```python
from build123d import *

# Parameters (mm, degrees)
SKETCH1_W           = 76.2
SKETCH1_H           = 76.2
SKETCH1_R           = 3.175
BOSS_EXTRUDE1_DEPTH = 6.35
SKETCH2_W           = 28.575
SKETCH2_H           = 76.2
SKETCH2_R           = 3.175
BOSS_EXTRUDE3_DEPTH = 9.525
SKETCH4_W           = 12.7
SKETCH4_H           = 25.4
CUT_EXTRUDE1_DEPTH  = 28.575
SKETCH5_W           = 12.7
SKETCH5_H           = 32.4
CUT_EXTRUDE2_DEPTH  = 9.525
SKETCH6_R           = 1
CUT_EXTRUDE3_DEPTH  = 6.35
SKETCH7_W           = 12.7
SKETCH7_H           = 3.5
SKETCH7_R           = 1
BOSS_EXTRUDE4_DEPTH = 11.43


with BuildPart() as part:
    # Sketch1 → Boss-Extrude1 (new body)
    with BuildSketch(Plane.XY):
        Rectangle(SKETCH1_W, SKETCH1_H)
        with Locations((-28.575, 19.525)):
            Circle(SKETCH1_R, mode=Mode.SUBTRACT)
        with Locations((28.575, 19.525)):
            Circle(SKETCH1_R, mode=Mode.SUBTRACT)
        with Locations((28.575, -19.525)):
            Circle(SKETCH1_R, mode=Mode.SUBTRACT)
        with Locations((-28.575, -19.525)):
            Circle(SKETCH1_R, mode=Mode.SUBTRACT)
    extrude(amount=BOSS_EXTRUDE1_DEPTH)

    # Sketch2 → Boss-Extrude3 (add)
    with BuildSketch(Plane(origin=(0, 0, 0), x_dir=(-1, 0, 0), z_dir=(0, 0, -1))):
        with Locations((-23.8125, 0)):
            Rectangle(SKETCH2_W, SKETCH2_H)
        with Locations((-28.575, -19.525)):
            Circle(SKETCH2_R, mode=Mode.SUBTRACT)
        with Locations((-28.575, 19.525)):
            Circle(SKETCH2_R, mode=Mode.SUBTRACT)
        with Locations((23.8125, 0)):
            Rectangle(SKETCH2_W, SKETCH2_H)
        with Locations((28.575, -19.525)):
            Circle(SKETCH2_R, mode=Mode.SUBTRACT)
        with Locations((28.575, 19.525)):
            Circle(SKETCH2_R, mode=Mode.SUBTRACT)
    extrude(amount=BOSS_EXTRUDE3_DEPTH)

    # Sketch4 → Cut-Extrude1 (cut)
    with BuildSketch(Plane.ZY.offset(-9.525)):
        Rectangle(SKETCH4_W, SKETCH4_H)
    extrude(amount=-CUT_EXTRUDE1_DEPTH, mode=Mode.SUBTRACT)

    # Sketch5 → Cut-Extrude2 (cut)
    with BuildSketch(Plane(origin=(0, 0, -9.525), x_dir=(-1, 0, 0), z_dir=(0, 0, -1))):
        with Locations((-19.05, 0)):
            Rectangle(SKETCH5_W, SKETCH5_H)
    extrude(amount=-CUT_EXTRUDE2_DEPTH, mode=Mode.SUBTRACT)

    # Sketch6 → Cut-Extrude3 (cut)
    with BuildSketch(Plane(origin=(0, 0, 0), x_dir=(-1, 0, 0), z_dir=(0, 0, -1))):
        with Locations((-19.05, 14.45)):
            Circle(SKETCH6_R)
        with Locations((-19.05, -14.45)):
            Circle(SKETCH6_R)
    extrude(amount=-CUT_EXTRUDE3_DEPTH, mode=Mode.SUBTRACT)

    # Sketch7 → Boss-Extrude4 (add)
    with BuildSketch(Plane(origin=(0, 0, 0), x_dir=(-1, 0, 0), z_dir=(0, 0, -1))):
        with Locations((-19.05, -14.45)):
            Rectangle(SKETCH7_W, SKETCH7_H)
        with Locations((-19.05, -14.45)):
            Circle(SKETCH7_R, mode=Mode.SUBTRACT)
        with Locations((-19.05, 14.45)):
            Rectangle(SKETCH7_W, SKETCH7_H)
        with Locations((-19.05, 14.45)):
            Circle(SKETCH7_R, mode=Mode.SUBTRACT)
    extrude(amount=BOSS_EXTRUDE4_DEPTH)


solid = part.part
```
Here's how the part is built. I have some questions about the finished solid (model axes, mm). A direction names the side the tool comes from. Coordinates: 2 decimals unless noted, no trailing zeros. Write each loop counter-clockwise with the first axis right and the second up, starting at its lowest first coordinate (ties: lowest second). Pieces come first, ordered by that corner, then holes. Notation, with made-up numbers: (13.5, 54) -> (45.5, 54) arc R15 ccw to (45.5, 59) -> close; hole circle Ø4 at (-33, -24). An arc over 180 degrees is marked (long way). Use a Markdown table: item, result. Add a question column.
(1) I'm going to push flat-ended pins straight in: P1, Ø1.5, axis at y = -14.5, z = -11, coming from the -X side; P2, Ø0.6, axis at x = 16.5, z = -10.5, coming from the -Y side; P3, Ø8.5, axis at x = 28.575, y = -19.525, coming from the -Z side (3 decimals). Where does each tip first touch, or does it pass through?
(2) For faces 1 (the flat face through (12.7, 14, -10)), 2 (the flat face through (32, 0, -6.35)), 3 (the flat face through (19, -16.2, -10)), 4 (the flat face through (25.4, 14, -10)), which set-ups out of +Z, -Z, +X, -X, +Y, -Y let a thin tool reach every point of the face, with its end or its side?
(3) Please list where these lines run through material, in increasing order: line 1 (Y direction, x = 19.05, z = -4); line 2 (Y direction, x = -28.5, z = 2.25); line 3 (Y direction, x = 14, z = 0.25).
(4) If we section it at D-D, the plane y = -14.45: Write out the boundary of the cut face in (x, z) (3 decimals).
(5) We'd pull the mould along Y, two halves only. Please class faces 5 (the flat face through (-9.525, -1, -5)), 6 (the flat face through (19, 16.2, -10)), 7 (the flat face through (25.4, 0, -8)): +Y half, -Y half, draft (parallel to the pull), parting line (faces both ways), or undercut.
(6) If we section it at C-C, the plane x = 19.05: Write out the boundary of the cut face in (y, z) (3 decimals), and give its area (3 significant figures).
(7) If we section it at B-B, the plane y = 5.5: Write out the boundary of the cut face in (x, z) (3 decimals), and give its area (3 significant figures).
(8) If we section it at A-A, the plane z = -10.5: Write out the boundary of the cut face in (x, y).
Outcome:
| question | item | result |
|---|---|---|
| 1 | P1 | stops at x = 12.7 |
| 1 | P2 | stops at y = -16.2 |
| 1 | P3 | stops at z = -9.525 |
| 2 | face 1 | -Z, -X, +Y, -Y |
| 2 | face 2 | +Z, +X |
| 2 | face 3 | -Z, +X, -X, -Y |
| 2 | face 4 | -Z, +X, +Y, -Y |
| 3 | line 1 | y = -38.1 to -15.45, -13.45 to -12.7, 12.7 to 13.45, 15.45 to 38.1 |
| 3 | line 2 | y = -38.1 to -22.7, -16.35 to 16.35, 22.7 to 38.1 |
| 3 | line 3 | y = -38.1 to -12.7, 12.7 to 38.1 |
| 4 | outline | (-38.1, -9.525) -> (-9.525, -9.525) -> (-9.525, 0) -> (9.525, 0) -> (9.525, -9.525) -> (12.7, -9.525) -> (12.7, -11.43) -> (18.05, -11.43) -> (18.05, 6.35) -> (-38.1, 6.35) -> close; (20.05, -11.43) -> (25.4, -11.43) -> (25.4, -9.525) -> (38.1, -9.525) -> (38.1, 6.35) -> (20.05, 6.35) -> close |
| 5 | face 5 | draft |
| 5 | face 6 | +Y half |
| 5 | face 7 | undercut |
| 6 | outline | (-38.1, -9.525) -> (-16.2, -9.525) -> (-16.2, -11.43) -> (-15.45, -11.43) -> (-15.45, 6.35) -> (-38.1, 6.35) -> close; (-13.45, -11.43) -> (-12.7, -11.43) -> (-12.7, 6.35) -> (-13.45, 6.35) -> close; (12.7, -11.43) -> (13.45, -11.43) -> (13.45, 6.35) -> (12.7, 6.35) -> close; (15.45, -11.43) -> (16.2, -11.43) -> (16.2, -9.525) -> (38.1, -9.525) -> (38.1, 6.35) -> (15.45, 6.35) -> close |
| 6 | area | 749 mm^2 |
| 7 | outline | (-38.1, -9.525) -> (-9.525, -9.525) -> (-9.525, 0) -> (9.525, 0) -> (9.525, 6.35) -> (-38.1, 6.35) -> close; (9.525, -9.525) -> (12.7, -9.525) -> (12.7, -6.35) -> (9.525, -6.35) -> close; (25.4, -9.525) -> (38.1, -9.525) -> (38.1, -6.35) -> (25.4, -6.35) -> close |
| 7 | area | 625 mm^2 |
| 8 | outline | (12.7, -16.2) -> (25.4, -16.2) -> (25.4, -12.7) -> (12.7, -12.7) -> close; (12.7, 12.7) -> (25.4, 12.7) -> (25.4, 16.2) -> (12.7, 16.2) -> close; hole circle Ø2 at (19.05, -14.45); hole circle Ø2 at (19.05, 14.45) |
